Work out the finished part from the listing and answer in its coordinate system (mm). A direction names the side the tool comes from. Coordinates: 2 decimals unless noted, no trailing zeros. Order: outer loops, then holes, each group sorted by start corner. A loop starts at its lowest first (then second) coordinate and runs counter-clockwise, first axis right, second up. Notation, with made-up numbers: (-14, 31) - (39, 31) arc R18 cw to (39, 49) - close; hole circle Ø9 at (66.25, 12.25). An arc over 180 degrees is marked (long way). Answer as a JSON object with one key per item and string values. Group by question number.
1) Section C-C (x = 13) is taken. Give the vertices of the cut face in (y, z).
2) Section A-A (y = 3.5) is taken. Give the vertices of the cut face in (x, z).
3) Each of these flat-tipped pins is pushed along its axis until it touches: P1, Ø1.5, axis at x = 10, y = 4.5, coming from the -Z side; P2, Ø1.8, axis at x = -11.5, z = 8, coming from the -Y side; P3, Ø4.5, axis at x = 14, z = 9, coming from the -Y side; P4, Ø2, axis at y = 1, z = 7, coming from the -X side. Where does it stop, or does it pass through?
4) Section B-B (y = -6.75) is taken. Give the vertices of the cut face in (x, z), plus the area to 3 significant figures.
5) A tool of negligible diameter and unlimited length cuts with its end or side. For faces 1 (the face through (-13, 8.5, 10)), 2 (the face through (-7.694, 9.719, 10.14)), 3 (the face through (-29, -8.5, 10)), from which of +Z, -Z, +X, -X, +Y, -Y can it reach the whole face along a straight path? Write none if from no direction.
6) Find the intervals of material crossed by line 1 along X through (y, z) = (5.5, 11); line 2 along X through (y, z) = (1.25, 4.5) (3 decimals); line 3 along Y through (x, z) = (11.5, 9.25), in increasing order.
7) The mould has two halves that part along X. Classify faces 4 (the face through (29, -8.5, 10)), 5 (the face through (19.885, -0.633, 9.86)), 6 (the face through (24.62, -8.26, 10.14)): released by +X, released by -X, zero draft, split by the parting line, or undercut.
8) Section D-D (x = -21.5) is taken. Give the vertices of the cut face in (y, z).
from build123d import *

# Parameters (mm, degrees)
F1_DEPTH = 20
F2_R     = 1.3846892623
F3_R     = 0.6428654195


# Not quite as in the source:
# - a feature names something its author has since deleted; it is built from what else it names


with BuildPart() as f1:
    # F0 (on Top) → F1 (new body)
    with BuildSketch(Plane.XY):
        Polygon((0, -1.5), (0, 0), (-4.5, 0), (-7.5, 10), (-17.5, 10), (-24.4375, -8.5), (-33.3979992978, -8.5), (-33.3979992978, -10), (-25, -10), (-23.3979992978, -10), (-16.4604992978, 8.5), (-8.6160459763, 8.5), (-5.6160459763, -1.5), align=None)
        Polygon((4.5, 0), (0, 0), (0, -1.5), (5.6160459763, -1.5), (8.6160459763, 8.5), (16.4604992978, 8.5), (23.3979992978, -10), (33.3979992978, -10), (33.3979992978, -8.5), (24.4375, -8.5), (17.5, 10), (7.5, 10), align=None)
    extrude(amount=F1_DEPTH)

    # F2
    f2_edges = [f1.edges().sort_by_distance(p)[0] for p in [
        (-7.5, 10, 10),
        (-4.5, 0, 10),
        (-17.5, 10, 10),
        (-16.460499, 8.5, 10),
        (-8.616046, 8.5, 10),
        (-5.616046, -1.5, 10),
        (17.5, 10, 10),
        (7.5, 10, 10),
        (4.5, 0, 10),
        (24.4375, -8.5, 10),
        (-24.4375, -8.5, 10),
        (5.616046, -1.5, 10),
        (8.616046, 8.5, 10),
        (16.460499, 8.5, 10),
        (23.397999, -10, 10),
        (-23.397999, -10, 10),
    ]]
    fillet(f2_edges, radius=F2_R)

    # F3
    f3_edges = [f1.edges().sort_by_distance(p)[0] for p in [
        (-33.397999, -8.5, 10),
        (33.397999, -8.5, 10),
    ]]
    fillet(f3_edges, radius=F3_R)


solid = f1.part
Report:
{
 "1": {"outline": "(8.5, 0) - (10, 0) - (10, 20) - (8.5, 20) - close"},
 "2": {"outline": "(-19.94, 0) - (-18.34, 0) - (-18.34, 20) - (-19.94, 20) - close; (-7.12, 0) - (-5.55, 0) - (-5.55, 20) - (-7.12, 20) - close; (5.55, 0) - (7.12, 0) - (7.12, 20) - (5.55, 20) - close; (18.34, 0) - (19.94, 0) - (19.94, 20) - (18.34, 20) - close"},
 "3": {"P1": "passes through", "P2": "stops at y = 8.5", "P3": "stops at y = 8.28", "P4": "stops at x = -21.25"},
 "4": {"outline": "(-23.78, 0) - (-22.18, 0) - (-22.18, 20) - (-23.78, 20) - close; (22.18, 0) - (23.78, 0) - (23.78, 20) - (22.18, 20) - close", "area": "64.1 mm²"},
 "5": {"face 1": "+Z, -Z, -Y", "face 2": "+Z, -Z, +Y", "face 3": "+Z, -Z, -X, +Y"},
 "6": {"line 1": "x = -19.19 to -17.59, -7.72 to -6.15, 6.15 to 7.72, 17.59 to 19.19", "line 2": "x = -20.781 to -19.179, -6.441 to -4.875, 4.875 to 6.441, 19.179 to 20.781", "line 3": "y = 8.5 to 10"},
 "7": {"face 4": "zero draft", "face 5": "undercut", "face 6": "released by +X"},
 "8": {"outline": "(-4.94, 0) - (-0.67, 0) - (-0.67, 20) - (-4.94, 20) - close"}
}
